For this review, take the finished solid that the model builds, in its own axes (mm). Face numbers are marked on the shaded views. A direction names the side the tool comes from. Give positions to 0.01 mm unless a question says otherwise; leave off trailing zeros. Loops run counter-clockwise (first coordinate to the right, second up) from the corner with the lowest first, then second, coordinate; pieces in that order, holes last. Notation, with made-up numbers: (-28, 36.5) -> (0, 36.5) arc R36 cw to (0, 75.5) -> close; hole circle Ø11 at (-32.5, 73.5). An arc over 180 degrees is marked (long way). Answer as CSV lines item,"result". Start each with the question number.
Item 1: Add section C-C on x = 0. State the section outline as (y, z) points.
Item 2: For L1, parallel to X at y = -90, z = 0; L2, parallel to Z at x = 4.5, y = -25; L3, parallel to X at y = 28, z = 14.5, list the stretches that pass through material, from the lowest coordinate up. Write a range as from..to.
Item 3: Machinability: for the marked faces 4, 5, 6, 7 and 8, which of the approach directions +Z, -Z, +X, -X, +Y, -Y give a long, thin tool a straight path to every point of the face, cutting with its end or side? Answer none if there is none.
Item 4: Add section B-B on z = 148. State the section outline as (x, y) points, plus the area to 3 significant figures.
Item 5: Add section A-A on x = -87.5. State how many separate pieces and enclosed holes the cut face has, plus the area to 3 significant figures.
Item 6: Add section D-D on y = 0. State the section outline as (x, z) points, plus the area to 3 significant figures.
Item 7: Clearance check with flat-ended pins moving along their axes: P1, Ø10, axis at y = -39, z = 68.5, coming from the -X side; P2, Ø1, axis at x = 123.5, y = -38, coming from the +Z side; P3, Ø3, axis at x = 14.5, y = -8.5, coming from the -Z side. State where each tip first meets the part, or that it passes through.
Item 8: The part is to be moulded in two halves that separate along X. For the marked faces 1, 2 and 3, say which applies: +X half, -X half, draft (parallel to the pull), parting line (faces both ways), or undercut.
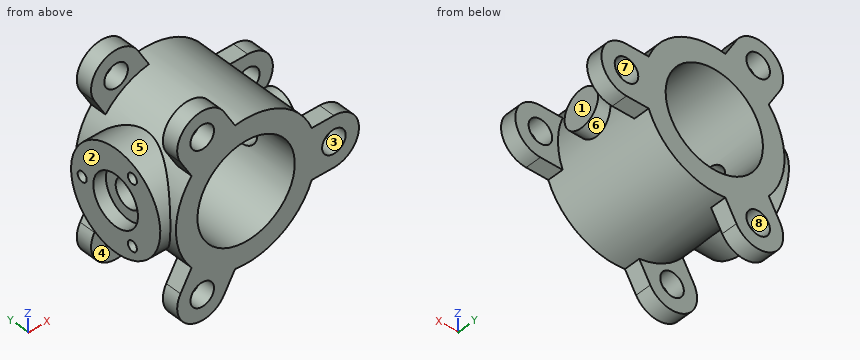
```python
from build123d import *

# Parameters (mm, degrees)
SKETCH1_R                = 140
SKETCH1_R_2              = 97
BOSS_EXTRUDE1_DEPTH      = 112.5
SKETCH2_R                = 23.5
BOSS_EXTRUDE2_DEPTH      = 32
CIRPATTERN1_COUNT        = 3
MIRROR1_COPY_1_SKETCH_R  = 23.5
MIRROR1_COPY_1_DEPTH     = 32
MIRROR1_COPY_2_SKETCH_R  = 23.5
MIRROR1_COPY_2_DEPTH     = 32
BOSS_EXTRUDE3_REACH      = 450.894
BOSS_EXTRUDE3_END_RADIUS = 140
SKETCH7_R                = 100
SKETCH8_R                = 50
CUT_EXTRUDE1_DEPTH       = 25
BOSS_EXTRUDE4_REACH      = 400.629
BOSS_EXTRUDE4_END_RADIUS = 140
SKETCH10_R               = 37.5
SKETCH9_R                = 28.1
CUT_EXTRUDE2_DEPTH       = 285
SKETCH11_R               = 10.15
CUT_EXTRUDE3_DEPTH       = 15
CIRPATTERN2_COUNT        = 3


with BuildPart() as part:
    # Sketch1 → Boss-Extrude1 (new, symmetric)
    with BuildSketch(Plane(origin=(0, 0, 0), x_dir=(1, 0, 0), z_dir=(0, 1, 0))):
        with Locations(Location((0, 0, 0), (0, 0, 270))):
            Circle(SKETCH1_R)
        with Locations(Location((0, 0, 0), (0, 0, 270))):
            Circle(SKETCH1_R_2, mode=Mode.SUBTRACT)
    extrude(amount=BOSS_EXTRUDE1_DEPTH, both=True)

    # Sketch2 → Boss-Extrude2 (add)
    with BuildSketch(Plane(origin=(0, 112.5, 0), x_dir=(1, 0, 0), z_dir=(0, 1, 0))):
        with BuildLine():
            Line((175, 50), (130.766968306, 50))
            ThreePointArc((130.766968306, 50), (140, 0), (130.766968306, -50))
            Line((130.766968306, -50), (175, -50))
            ThreePointArc((175, -50), (225, 0), (175, 50))
        make_face()
        with Locations(Location((175, 0, 0), (0, 0, 270))):
            Circle(SKETCH2_R, mode=Mode.SUBTRACT)
    boss_extrude2 = extrude(amount=-BOSS_EXTRUDE2_DEPTH)

    # CirPattern1: Boss-Extrude2 ×3 about axis
    cirpattern1_axis = Axis((0, 0, 0), (0, 1, 0))
    for i in range(1, CIRPATTERN1_COUNT):
        add(boss_extrude2.rotate(cirpattern1_axis, i * 360 / CIRPATTERN1_COUNT))

    # Mirror1: Boss-Extrude2 across plane
    add(boss_extrude2.mirror(Plane.ZX))

    # Mirror1 copy 1 sketch → Mirror1 copy 1 (add)
    with BuildSketch(Plane(origin=(0, -112.5, 0), x_dir=(-0.4999999999999998, 0, -0.8660254037844387), z_dir=(0, -1, 0))):
        with BuildLine():
            Line((175, -50), (130.766968306, -50))
            ThreePointArc((130.766968306, -50), (140, 0), (130.766968306, 50))
            Line((130.766968306, 50), (175, 50))
            ThreePointArc((175, 50), (225, 0), (175, -50))
        make_face()
        with Locations((175, 0)):
            Circle(MIRROR1_COPY_1_SKETCH_R, mode=Mode.SUBTRACT)
    extrude(amount=-MIRROR1_COPY_1_DEPTH)

    # Mirror1 copy 2 sketch → Mirror1 copy 2 (add)
    with BuildSketch(Plane(origin=(0, -112.5, 0), x_dir=(-0.5000000000000004, 0, 0.8660254037844384), z_dir=(0, -1, 0))):
        with BuildLine():
            Line((175, -50), (130.766968306, -50))
            ThreePointArc((130.766968306, -50), (140, 0), (130.766968306, 50))
            Line((130.766968306, 50), (175, 50))
            ThreePointArc((175, 50), (225, 0), (175, -50))
        make_face()
        with Locations((175, 0)):
            Circle(MIRROR1_COPY_2_SKETCH_R, mode=Mode.SUBTRACT)
    extrude(amount=-MIRROR1_COPY_2_DEPTH)

    # Boss-Extrude3: up to this cylinder (the profile starts outside it)
    boss_extrude3_end = Plane(origin=(0, 0, 0), z_dir=(0, -1, 0)) * Cylinder(BOSS_EXTRUDE3_END_RADIUS, 1182.788, mode=Mode.PRIVATE)
    # Sketch7 → Boss-Extrude3 (add, up to the surface)
    with BuildSketch(Plane(origin=(-160, 0, 0), x_dir=(0, 0, -1), z_dir=(1, 0, 0)), mode=Mode.PRIVATE) as boss_extrude3_sk1:
        with Locations(Location((0, 0, 0), (0, 0, 180))):
            Circle(SKETCH7_R)
    boss_extrude3_tool1 = extrude(boss_extrude3_sk1.sketch, amount=BOSS_EXTRUDE3_REACH, mode=Mode.PRIVATE) - boss_extrude3_end
    add(boss_extrude3_tool1.solids().sort_by_distance((-160, 0, 0))[0])

    # Sketch8 → Cut-Extrude1 (cut)
    with BuildSketch(Plane.ZY.offset(160)):
        Circle(SKETCH8_R)
    extrude(amount=-CUT_EXTRUDE1_DEPTH, mode=Mode.SUBTRACT)

    # Boss-Extrude4: up to this cylinder (the profile starts outside it)
    boss_extrude4_end = Plane(origin=(0, 0, 0), z_dir=(0, -1, 0)) * Cylinder(BOSS_EXTRUDE4_END_RADIUS, 1082.258, mode=Mode.PRIVATE)
    # Sketch10 → Boss-Extrude4 (add, up to the surface)
    with BuildSketch(Plane(origin=(165, 0, 0), x_dir=(0, 0, -1), z_dir=(1, 0, 0)), mode=Mode.PRIVATE) as boss_extrude4_sk1:
        Circle(SKETCH10_R)
    boss_extrude4_tool1 = extrude(boss_extrude4_sk1.sketch, amount=-BOSS_EXTRUDE4_REACH, mode=Mode.PRIVATE) - boss_extrude4_end
    add(boss_extrude4_tool1.solids().sort_by_distance((165, 0, 0))[0])

    # Sketch9 → Cut-Extrude2 (cut)
    with BuildSketch(Plane.ZY.offset(135)):
        Circle(SKETCH9_R)
    extrude(amount=-CUT_EXTRUDE2_DEPTH, mode=Mode.SUBTRACT)

    # Sketch11 → Cut-Extrude3 (cut)
    with BuildSketch(Plane.ZY.offset(160)):
        with Locations((0, 75)):
            Circle(SKETCH11_R)
    cut_extrude3 = extrude(amount=-CUT_EXTRUDE3_DEPTH, mode=Mode.SUBTRACT)

    # CirPattern2: Cut-Extrude3 ×3 about axis
    cirpattern2_axis = Axis((0, 0, 0), (1, 0, 0))
    for i in range(1, CIRPATTERN2_COUNT):
        add(cut_extrude3.rotate(cirpattern2_axis, i * 360 / CIRPATTERN2_COUNT), mode=Mode.SUBTRACT)


solid = part.part
```
Computed values:
1,outline,"(-112.5, -140) -> (112.5, -140) -> (112.5, -97) -> (-112.5, -97) -> close; (-112.5, 97) -> (112.5, 97) -> (112.5, 140) -> (-112.5, 140) -> close"
2,L1,"-160..-97, 97..151.5, 198.5..225"
2,L2,"-139.93..-96.9, 96.9..139.93"
2,L3,"-135..-95.91, 95.91..165"
3,face 4,"-Z, -X"
3,face 5,"-X"
3,face 6,"+X"
3,face 7,"+Y"
3,face 8,"+Y, -Y"
4,outline,"(-137.37, -112.5) -> (-110.73, -112.5) -> (-110.73, -80.5) -> (-137.37, -80.5) -> close; (-137.37, 80.5) -> (-110.73, 80.5) -> (-110.73, 112.5) -> (-137.37, 112.5) -> close; (-64.27, -112.5) -> (-27.71, -112.5) -> (-27.71, -80.5) -> (-64.27, -80.5) -> close; (-64.27, 80.5) -> (-27.71, 80.5) -> (-27.71, 112.5) -> (-64.27, 112.5) -> close"
4,area,"4,040 mm²"
5,separate pieces,"6"
5,enclosed holes,"0"
5,area,"36,100 mm²"
6,outline,"(-160, -100) -> (-97.98, -100) arc R140 ccw to (134.88, -37.5) -> (165, -37.5) -> (165, 37.5) -> (134.88, 37.5) arc R140 ccw to (-97.98, 100) -> (-160, 100) -> (-160, 50) -> (-135, 50) -> (-135, 28.1) -> (-92.84, 28.1) arc R97 cw to (92.84, 28.1) -> (150, 28.1) -> (150, -28.1) -> (92.84, -28.1) arc R97 cw to (-92.84, -28.1) -> (-135, -28.1) -> (-135, -50) -> (-160, -50) -> close"
6,area,"32,900 mm²"
7,P1,"x = -145"
7,P2,"z = 66.87"
7,P3,"z = -139.4"
8,face 1,"+X half"
8,face 2,"-X half"
8,face 3,"undercut"
